from build123d import *

# Parameters (mm, degrees)
EXTRUDE_1_DEPTH       = 2.5
SKETCH_1_3_W          = 21.9
SKETCH_1_3_H          = 3
EXTRUDE_2_DEPTH       = 0.5
SKETCH_2_R            = 1
CUT_EXTRUDE_1_DEPTH   = 34.660057049
SKETCH_3_W            = 21.9
SKETCH_3_H            = 3
CUT_EXTRUDE_2_DEPTH   = 1.5
SKETCH_4_W            = 39.2
SKETCH_4_H            = 52.23
EXTRUDE_3_DEPTH       = 1
CUT_EXTRUDE_START     = -1
CUT_EXTRUDE_3_DEPTH   = 1
FILLET_1_R            = 4
CUT_EXTRUDE_1_2_DEPTH = 1
FILLET_2_R            = 5


with BuildPart() as part:
    # Sketch 1 → Extrude 1 (new body)
    with BuildSketch(Plane(origin=(0, 0, 0), x_dir=(1, 0, 0), z_dir=(0, 1, 0))):
        with BuildLine():
            ThreePointArc((13.158319986, 21.726795167), (16.799919909, 20.21839509), (18.308319986, 16.576795167))
            Line((18.308319986, 16.576795167), (18.308319986, 26.726795167))
            Line((18.308319986, 26.726795167), (13.158319986, 26.726795167))
            Line((13.158319986, 26.726795167), (13.158319986, 23.726795167))
            Line((13.158319986, 23.726795167), (-8.741680014, 23.726795167))
            Line((-8.741680014, 23.726795167), (-8.741680014, 26.726795167))
            Line((-8.741680014, 26.726795167), (-13.891680014, 26.726795167))
            Line((-13.891680014, 26.726795167), (-13.891680014, 16.576795167))
            ThreePointArc((-13.891680014, 16.576795167), (-12.383279937, 20.21839509), (-8.741680014, 21.726795167))
            Line((-8.741680014, 21.726795167), (13.158319986, 21.726795167))
        make_face()
        Polygon((-13.891680014, -22.503204833), (-13.891680014, -12.353204833), (-13.891680014, 16.576795167), (-13.891680014, 26.726795167), (-15.891680014, 26.726795167), (-15.891680014, -22.503204833), align=None)
        with BuildLine():
            ThreePointArc((13.158319986, -17.503204833), (16.799919909, -15.994804756), (18.308319986, -12.353204833))
            Line((18.308319986, -12.353204833), (18.308319986, -22.503204833))
            Line((18.308319986, -22.503204833), (-13.891680014, -22.503204833))
            Line((-13.891680014, -22.503204833), (-13.891680014, -12.353204833))
            ThreePointArc((-13.891680014, -12.353204833), (-12.383279937, -15.994804756), (-8.741680014, -17.503204833))
            Line((-8.741680014, -17.503204833), (13.158319986, -17.503204833))
        make_face()
        Polygon((18.308319986, 16.576795167), (18.308319986, -12.353204833), (18.308319986, -22.503204833), (20.308319986, -22.503204833), (20.308319986, 26.726795167), (18.308319986, 26.726795167), align=None)
    extrude(amount=EXTRUDE_1_DEPTH)

    # Sketch 1_3 → Extrude 2 (add)
    with BuildSketch(Plane(origin=(0, 0, 0), x_dir=(1, 0, 0), z_dir=(0, 1, 0))):
        with Locations((2.208319986, 25.226795167)):
            Rectangle(SKETCH_1_3_W, SKETCH_1_3_H)
    extrude(amount=EXTRUDE_2_DEPTH)

    # Sketch 2 → Cut-Extrude 1 (cut, through all)
    with BuildSketch(Plane.XZ):
        with Locations(Location((-11.891680014, -24.726795167, 0), (0, 0, 270))):
            Circle(SKETCH_2_R)
        with Locations(Location((-11.891680014, 20.503204833, 0), (0, 0, 270))):
            Circle(SKETCH_2_R)
        with Locations(Location((16.308319986, 20.503204833, 0), (0, 0, 270))):
            Circle(SKETCH_2_R)
        with Locations(Location((16.308319986, -24.726795167, 0), (0, 0, 270))):
            Circle(SKETCH_2_R)
    extrude(amount=-CUT_EXTRUDE_1_DEPTH, mode=Mode.SUBTRACT)

    # Sketch 3 → Cut-Extrude 2 (cut)
    with BuildSketch(Plane(origin=(0, 2.5, 0), x_dir=(1, 0, 0), z_dir=(0, 1, 0))):
        with Locations((2.208319986, -19.003204833)):
            Rectangle(SKETCH_3_W, SKETCH_3_H)
    extrude(amount=-CUT_EXTRUDE_2_DEPTH, mode=Mode.SUBTRACT)

    # Sketch 4 → Extrude 3 (add)
    with BuildSketch(Plane.XZ):
        with Locations((2.208319986, -2.111795167)):
            Rectangle(SKETCH_4_W, SKETCH_4_H)
    extrude(amount=EXTRUDE_3_DEPTH)

    # Sketch 5 → Cut-Extrude 3 (cut)
    with BuildSketch(Plane(origin=(0, 0, 0), x_dir=(1, 0, 0), z_dir=(0, 1, 0)).offset(CUT_EXTRUDE_START)):
        with BuildLine():
            Line((18.308319986, -12.353204833), (18.308319986, 16.576795167))
            ThreePointArc((18.308319986, 16.576795167), (16.799919909, 20.21839509), (13.158319986, 21.726795167))
            Line((13.158319986, 21.726795167), (-8.741680014, 21.726795167))
            ThreePointArc((-8.741680014, 21.726795167), (-12.383279937, 20.21839509), (-13.891680014, 16.576795167))
            Line((-13.891680014, 16.576795167), (-13.891680014, -12.353204833))
            ThreePointArc((-13.891680014, -12.353204833), (-12.383279937, -15.994804756), (-8.741680014, -17.503204833))
            Line((-8.741680014, -17.503204833), (13.158319986, -17.503204833))
            ThreePointArc((13.158319986, -17.503204833), (16.799919909, -15.994804756), (18.308319986, -12.353204833))
        make_face()
    extrude(amount=CUT_EXTRUDE_3_DEPTH, mode=Mode.SUBTRACT)

    # Fillet 1
    fillet_1_edges = [part.edges().sort_by_distance(p)[0] for p in [
        (-15.891680014, 1.25, 22.503204833),
        (-15.891680014, 1.25, -26.726795167),
        (20.308319986, 1.25, -26.726795167),
        (20.308319986, 1.25, 22.503204833),
    ]]
    fillet(fillet_1_edges, radius=FILLET_1_R)

    # Sketch 5_2 → Cut-Extrude 1 2 (cut)
    with BuildSketch(Plane(origin=(0, 0, 0), x_dir=(1, 0, 0), z_dir=(0, 1, 0)).offset(CUT_EXTRUDE_START)):
        with BuildLine():
            Line((-8.741680014, -18.003204833), (13.158319986, -18.003204833))
            ThreePointArc((13.158319986, -18.003204833), (17.153473299, -16.348358147), (18.808319986, -12.353204833))
            Line((18.808319986, -12.353204833), (18.808319986, 16.576795167))
            ThreePointArc((18.808319986, 16.576795167), (17.153473299, 20.571948481), (13.158319986, 22.226795167))
            Line((13.158319986, 22.226795167), (-8.741680014, 22.226795167))
            ThreePointArc((-8.741680014, 22.226795167), (-12.736833328, 20.571948481), (-14.391680014, 16.576795167))
            Line((-14.391680014, 16.576795167), (-14.391680014, -12.353204833))
            ThreePointArc((-14.391680014, -12.353204833), (-12.736833328, -16.348358147), (-8.741680014, -18.003204833))
        make_face()
        with BuildLine():
            Line((-8.741680014, -17.503204833), (13.158319986, -17.503204833))
            ThreePointArc((13.158319986, -17.503204833), (16.799919909, -15.994804756), (18.308319986, -12.353204833))
            Line((18.308319986, -12.353204833), (18.308319986, 16.576795167))
            ThreePointArc((18.308319986, 16.576795167), (16.799919909, 20.21839509), (13.158319986, 21.726795167))
            Line((13.158319986, 21.726795167), (-8.741680014, 21.726795167))
            ThreePointArc((-8.741680014, 21.726795167), (-12.383279937, 20.21839509), (-13.891680014, 16.576795167))
            Line((-13.891680014, 16.576795167), (-13.891680014, -12.353204833))
            ThreePointArc((-13.891680014, -12.353204833), (-12.383279937, -15.994804756), (-8.741680014, -17.503204833))
        make_face(mode=Mode.SUBTRACT)
    extrude(amount=CUT_EXTRUDE_1_2_DEPTH, mode=Mode.SUBTRACT)

    # Fillet 2
    fillet_2_edges = [part.edges().sort_by_distance(p)[0] for p in [
        (21.808319986, -0.5, -28.226795167),
        (21.808319986, -0.5, 24.003204833),
        (-17.391680014, -0.5, 24.003204833),
        (-17.391680014, -0.5, -28.226795167),
    ]]
    fillet(fillet_2_edges, radius=FILLET_2_R)


solid = part.part
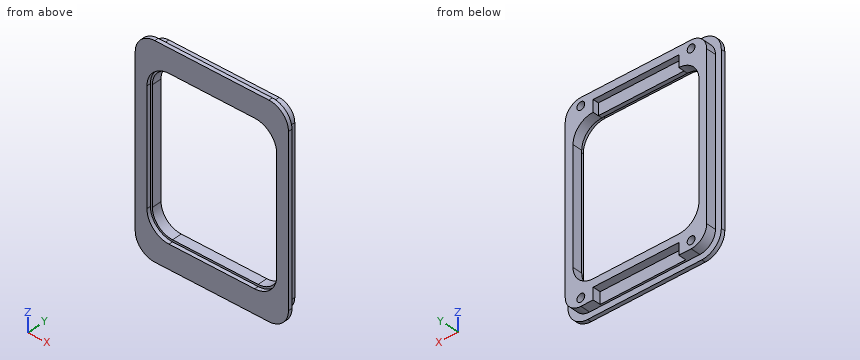
Work out the finished part from the listing and answer in its coordinate system (mm). Coordinates: 2 decimals unless noted, no trailing zeros. Write each loop counter-clockwise with the first axis right and the second up, starting at its lowest first coordinate (ties: lowest second). Pieces come first, ordered by that corner, then holes. Notation, with made-up numbers: (14, 75.25) - (63, 75.25) arc R30 cw to (63, 113.25) - close; hole circle Ø6 at (62.25, -34.75). An arc over 180 degrees is marked (long way). One line per question, with ' | ' between items.
1) Find section A-A, the plane x = 11.5. Determine the outline of the cut face in (y, z), and give its area (3 significant figures).
Checks:
outline: (-1, -28.23) - (0, -28.23) - (0, -26.73) - (0.5, -26.73) - (0.5, -23.73) - (2.5, -23.73) - (2.5, -21.73) - (0, -21.73) - (0, -22.23) - (-1, -22.23) - close; (-1, 18) - (0, 18) - (0, 17.5) - (1, 17.5) - (1, 20.5) - (2.5, 20.5) - (2.5, 22.5) - (0, 22.5) - (0, 24) - (-1, 24) - close | area: 26.5 mm2
2) Find section C-C, the plane y = 1.6. Determine the outline of the cut face in (x, z), and give its area (3 significant figures).
Checks:
outline: (-15.89, -22.73) arc R4 ccw to (-11.89, -26.73) - (-8.74, -26.73) - (-8.74, -23.73) - (13.16, -23.73) - (13.16, -26.73) - (16.31, -26.73) arc R4 ccw to (20.31, -22.73) - (20.31, 18.5) arc R4 ccw to (16.31, 22.5) - (-11.89, 22.5) arc R4 ccw to (-15.89, 18.5) - close; hole (-13.89, -16.58) arc R5.15 ccw to (-8.74, -21.73) - (13.16, -21.73) arc R5.15 ccw to (18.31, -16.58) - (18.31, 12.35) arc R5.15 ccw to (13.16, 17.5) - (13.16, 20.5) - (-8.74, 20.5) - (-8.74, 17.5) arc R5.15 ccw to (-13.89, 12.35) - close; hole circle Ø2 at (-11.89, -24.73); hole circle Ø2 at (-11.89, 20.5); hole circle Ø2 at (16.31, -24.73); hole circle Ø2 at (16.31, 20.5) | area: 384 mm2
3) Consider probe 1 along X at (y, z) = (1, 2.5); probe 2 along Z at (x, y) = (8.5, 1.6); probe 3 along Z at (x, y) = (-7, 0.3). Determine where each line is inside the solid, lowest interval first. Write a range as [from, to].
Checks:
probe 1: [-15.89, -13.89], [18.31, 20.31] | probe 2: [-23.73, -21.73], [20.5, 22.5] | probe 3: [-26.73, -21.73], [17.5, 22.5]
4) Find section B-B, the plane z = 7.5. Determine the outline of the cut face in (x, y), and give its area (3 significant figures).
Checks:
outline: (-17.39, -1) - (-14.39, -1) - (-14.39, 0) - (-13.89, 0) - (-13.89, 2.5) - (-15.89, 2.5) - (-15.89, 0) - (-17.39, 0) - close; (18.31, 0) - (18.81, 0) - (18.81, -1) - (21.81, -1) - (21.81, 0) - (20.31, 0) - (20.31, 2.5) - (18.31, 2.5) - close | area: 16.0 mm2
5) Find section D-D, the plane z = 13. Determine the outline of the cut face in (x, y), and give its area (3 significant figures).
Checks:
outline: (-17.39, -1) - (-14.35, -1) - (-14.35, 0) - (-13.85, 0) - (-13.85, 2.5) - (-15.89, 2.5) - (-15.89, 0) - (-17.39, 0) - close; (18.27, 0) - (18.77, 0) - (18.77, -1) - (21.81, -1) - (21.81, 0) - (20.31, 0) - (20.31, 2.5) - (18.27, 2.5) - close | area: 16.3 mm2
6) Flat-ended cylindrical pins translate along their axes: P1, Ø1.5, axis at x = -13, y = 1, coming from the -Z side; P2, Ø1.2, axis at y = 1.5, z = 4, coming from the +X side; P3, Ø1.5, axis at x = 0.5, z = 19, coming from the +Y side. Find the tip coordinate at first contact, or state that the pin passes through.
Checks:
P1: z = -26.71 | P2: x = 20.31 | P3: y = 1
